```python
from build123d import *

# Parameters (mm, degrees)
BOSS_EXTRUDE1_DEPTH = 100
BOSS_EXTRUDE2_DEPTH = 15
SKETCH3_W           = 20
SKETCH3_H           = 15
BOSS_EXTRUDE3_DEPTH = 60
SKETCH4_W           = 40
SKETCH4_H           = 33
CUT_EXTRUDE1_DEPTH  = 119.5
CUT_EXTRUDE2_DEPTH  = 119.5


with BuildPart() as part:
    # Sketch1 → Boss-Extrude1 (new body)
    with BuildSketch(Plane(origin=(0, 0, 0), x_dir=(1, 0, 0), z_dir=(0, 1, 0))):
        with BuildLine():
            Line((0, 0), (0, 15))
            Line((0, 15), (-20, 15))
            ThreePointArc((-20, 15), (-27.071067812, 17.928932188), (-30, 25))
            Line((-30, 25), (-30, 81))
            ThreePointArc((-30, 81), (-75.256322222, 31.603413808), (-40, -25.362796982))
            Line((-40, -25.362796982), (-40, 0))
            Line((-40, 0), (0, 0))
        make_face()
    extrude(amount=BOSS_EXTRUDE1_DEPTH)

    # Sketch2 → Boss-Extrude2 (add)
    with BuildSketch(Plane(origin=(0, 100, 0), x_dir=(1, 0, 0), z_dir=(0, 1, 0))):
        with BuildLine():
            Line((0, 5), (-75.235044142, 20.9917023))
            ThreePointArc((-75.235044142, 20.9917023), (-64.184418834, -7.177185713), (-40, -25.362796982))
            Line((-40, -25.362796982), (-40, 0))
            Line((-40, 0), (0, 0))
            Line((0, 0), (0, 5))
        make_face()
    extrude(amount=BOSS_EXTRUDE2_DEPTH)

    # Sketch3 → Boss-Extrude3 (add, symmetric)
    with BuildSketch(Plane(origin=(0, 50, 0), x_dir=(1, 0, 0), z_dir=(0, 1, 0))):
        with Locations((-35, 58.5)):
            Rectangle(SKETCH3_W, SKETCH3_H)
    extrude(amount=BOSS_EXTRUDE3_DEPTH, both=True)

    # Sketch4 → Cut-Extrude1 (cut, symmetric)
    with BuildSketch(Plane(origin=(0, 0, 0), x_dir=(0, 0, -1), z_dir=(1, 0, 0))):
        with Locations((61, 53.5)):
            Rectangle(SKETCH4_W, SKETCH4_H)
    extrude(amount=CUT_EXTRUDE1_DEPTH, both=True, mode=Mode.SUBTRACT)

    # Sketch5 → Cut-Extrude2 (cut, symmetric)
    with BuildSketch(Plane(origin=(0, 0, -15), x_dir=(-1, 0, 0), z_dir=(0, 0, -1))):
        with BuildLine():
            Line((15, 90), (15, 10))
            ThreePointArc((15, 10), (10, 5), (5, 10))
            Line((5, 10), (5, 90))
            ThreePointArc((5, 90), (10, 95), (15, 90))
        make_face()
    extrude(amount=CUT_EXTRUDE2_DEPTH, both=True, mode=Mode.SUBTRACT)


solid = part.part
```
Could you check a few things on this model? Use its own coordinates, in mm. A direction names the side the tool comes from. Coordinates: 2 decimals unless noted, no trailing zeros. Write each loop counter-clockwise with the first axis right and the second up, starting at its lowest first coordinate (ties: lowest second). Pieces come first, ordered by that corner, then holes. Notation, with made-up numbers: (-33.75, 45.25) -> (16.25, 45.25) arc R22 ccw to (16.25, 84.25) -> close; hole circle Ø4 at (-36, 30). An arc over 180 degrees is marked (long way). One line per question, with ' | ' between items. Start each with the question number.
1. Please list where these lines run through material, in increasing order: line 1 along Z through (x, y) = (-6, 3.5); line 2 along Y through (x, z) = (-37, -19.5); line 3 along Z through (x, y) = (-41.5, -0.5).
2. If we section it at D-D (z = 16): Please give me the cut outline in (x, y), and give its area (3 significant figures).
3. For faces 1 (the face through (-45, -5, -58)), 2 (the face through (-10, 95, -8)), 3 (the face through (-3, 49, -15)), which set-ups out of +Z, -Z, +X, -X, +Y, -Y let a thin tool reach every point of the face, with its end or its side?
4. If we section it at C-C (z = -69.5): Please give me the cut outline in (x, y), and give its area (3 significant figures).
5. Will these pins go through, and if not, where does the flat tip stop? P1, Ø7.5, axis at y = 84.5, z = -59, coming from the +X side; P2, Ø2, axis at x = -37, z = -48.5, coming from the +Y side; P3, Ø6, axis at x = -38, y = 8.5, coming from the -Z side.
6. Thinking about a two-plate mould opening in X: for faces 4 (the face through (-15, 51, -8)), 5 (the face through (-47, 100, -35)), 6 (the face through (-30, 18, -73)), which applies, pulls with the +X half, pulls with the -X half, needs draft (parallel to the pull), parting line crosses it, or undercut?
7. If we section it at A-A (y = 33.5): Please give me the cut outline in (x, z).
8. If we section it at B-B (x = -10): Please give me the cut outline in (y, z).
Return value:
1) line 1: z = -15 to 0 | line 2: y = 0 to 100 | line 3: z = -66 to -51
2) outline: (-55.8, 0) -> (-40, 0) -> (-40, 115) -> (-55.8, 115) -> close | area: 1,820 mm²
3) face 1: +Z, -Z, -X, -Y | face 2: +Z, -Z | face 3: -Z, +X, +Y, -Y
4) outline: (-54.98, 0) -> (-30, 0) -> (-30, 37) -> (-54.98, 37) -> close; (-54.98, 70) -> (-30, 70) -> (-30, 100) -> (-54.98, 100) -> close | area: 1,670 mm²
5) P1: stops at x = -25 | P2: stops at y = 100 | P3: stops at z = -79.84
6) face 4: undercut | face 5: needs draft | face 6: pulls with the +X half
7) outline: (-40, 0) -> (-40, 25.36) arc R55.5 ccw to (-30, -81) -> (-30, -66) -> (-25, -66) -> (-25, -51) -> (-30, -51) -> (-30, -25) arc R10 cw to (-20, -15) -> (-15, -15) -> (-15, 0) -> close; (-5, -15) -> (0, -15) -> (0, 0) -> (-5, 0) -> close
8) outline: (0, -15) -> (5, -15) -> (5, 0) -> (0, 0) -> close; (95, -15) -> (100, -15) -> (100, -7.13) -> (115, -7.13) -> (115, 0) -> (95, 0) -> close
